Job drawing, mm, ordinate dimensions from the low corner. One solid piece. Coordinates: 2 decimals unless noted, no trailing zeros. Loops run counter-clockwise (first coordinate to the right, second up) from the corner with the lowest first, then second, coordinate; pieces in that order, holes last. Notation, with made-up numbers: (-37, -37.75) -> (-24, -37.75) arc R12 cw to (-24, -31.75) -> close; hole circle Ø2 at (47, -14). An arc over 180 degrees is marked (long way). Use one line per item in the form item = value. Start each with the question number.
(1) Band-saw the part on C-C on y = 1.3. Give the cut face in (x, z), then the cut area to 3 significant figures.
(2) Band-saw the part on B-B on z = 32. Give the cut face in (x, y), then the cut area to 3 significant figures.
(3) Band-saw the part on A-A on x = 330.5. Give the cut face in (y, z).
(4) Drill centre lines: L1, parallel to Z at x = 52, y = 3; L2, parallel to X at y = 3.65, z = 24; L3, parallel to X at y = 3.05, z = 53. Where is each one in solid material? Low to high. Write a range as [from, to].
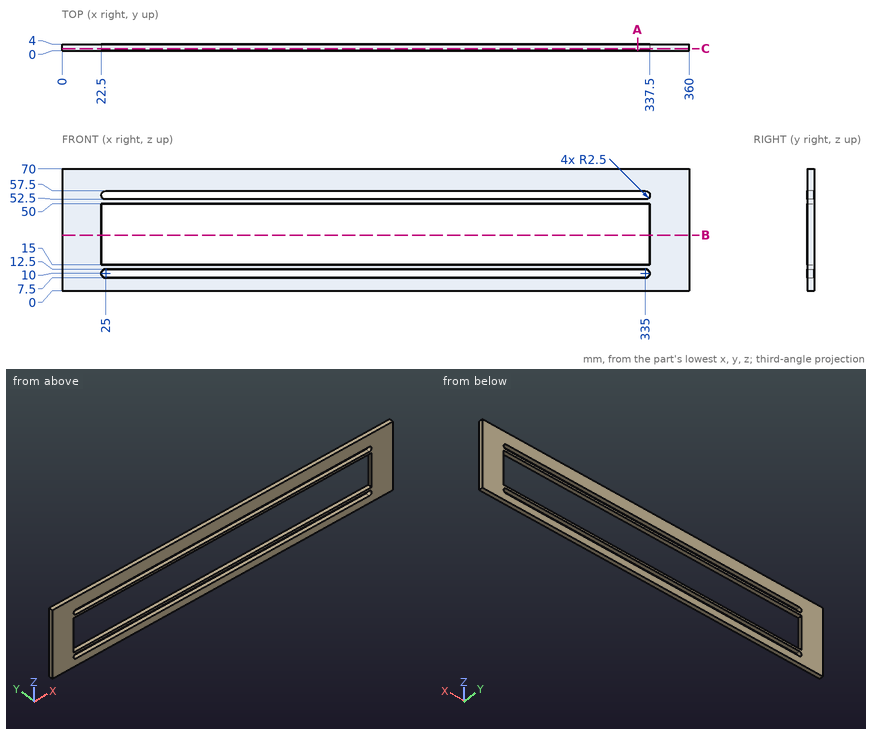
A:
q1.outline = (0, 0) -> (360, 0) -> (360, 70) -> (0, 70) -> close; hole (22.5, 15) -> (337.5, 15) -> (337.5, 50) -> (22.5, 50) -> close; hole (25, 7.5) -> (335, 7.5) arc R2.5 ccw to (335, 12.5) -> (25, 12.5) arc R2.5 ccw to start; hole (25, 52.5) -> (335, 52.5) arc R2.5 ccw to (335, 57.5) -> (25, 57.5) arc R2.5 ccw to start
q1.area = 11,000 mm²
q2.outline = (0, 0) -> (22.5, 0) -> (22.5, 4) -> (0, 4) -> close; (337.5, 0) -> (360, 0) -> (360, 4) -> (337.5, 4) -> close
q2.area = 180 mm²
q3.outline = (0, 0) -> (4, 0) -> (4, 7.5) -> (0, 7.5) -> close; (0, 12.5) -> (4, 12.5) -> (4, 15) -> (0, 15) -> close; (0, 50) -> (4, 50) -> (4, 52.5) -> (0, 52.5) -> close; (0, 57.5) -> (4, 57.5) -> (4, 70) -> (0, 70) -> close
q4.L1 = [0, 7.5], [12.5, 15], [50, 52.5], [57.5, 70]
q4.L2 = [0, 22.5], [337.5, 360]
q4.L3 = [0, 23.5], [336.5, 360]
